```python
from build123d import *

# Parameters (mm, degrees)
SKETCH2_W             = 67.071067812
SKETCH2_H             = 337.071067812
SKETCH2_W_2           = 60
SKETCH2_H_2           = 330
BOSS_EXTRUDE1_DEPTH   = 12.5
SKETCH3_W             = 67.071067812
SKETCH3_H             = 337.071067812
BOSS_EXTRUDE2_DEPTH   = 5
BODY_MOVE_COPY2_ANGLE = 180
BOSS_EXTRUDE3_DEPTH   = 5


with BuildPart() as part:
    # Sketch2 → Boss-Extrude1 (new body)
    with BuildSketch(Plane(origin=(0, 0, 0), x_dir=(1, 0, 0), z_dir=(0, 1, 0))):
        with Locations((30, 165)):
            Rectangle(SKETCH2_W, SKETCH2_H)
        with Locations((30, 165)):
            Rectangle(SKETCH2_W_2, SKETCH2_H_2, mode=Mode.SUBTRACT)
    extrude(amount=BOSS_EXTRUDE1_DEPTH)

    # Sketch3 → Boss-Extrude2 (add)
    with BuildSketch(Plane.XZ):
        with Locations((30, -165)):
            Rectangle(SKETCH3_W, SKETCH3_H)
    extrude(amount=BOSS_EXTRUDE2_DEPTH)


with BuildPart() as body_2:
    # Split1: the piece on the far side of the plane
    add(part.part)
    split(bisect_by=Plane(origin=(0, 0, -165), x_dir=(-1, 0, 0), z_dir=(0, 0, -1)), keep=Keep.BOTTOM)


with BuildPart() as part_1:
    add(part.part)

    # Split1
    split(bisect_by=Plane(origin=(0, 0, -165), x_dir=(-1, 0, 0), z_dir=(0, 0, -1)), keep=Keep.TOP)

    # Sketch4 → Boss-Extrude3 (add)
    with BuildSketch(Plane.XY.offset(-165)):
        Polygon((60, 0), (0, 0), (0, 12.5), (-3.535533906, 12.5), (-3.535533906, -5), (63.535533906, -5), (63.535533906, 12.5), (60, 12.5), align=None)
    extrude(amount=BOSS_EXTRUDE3_DEPTH)


with BuildPart() as body_2_1:
    # Body-Move/Copy2: read off the stored shape, not the designer's step
    # Body-Move/Copy2: moved
    add(body_2.part.moved(Location((-127.0710678, -25, 0))).rotate(Axis((0, 0, 0), (0, 0, 1)), BODY_MOVE_COPY2_ANGLE))


solid = part_1.part
```
Check sheet for the modelled part. Datum: model origin and axes. Units: mm. A direction names the side the tool comes from. Give positions to 0.01 mm unless a question says otherwise; leave off trailing zeros. Write each loop counter-clockwise with the first axis right and the second up, starting at its lowest first coordinate (ties: lowest second). Pieces come first, ordered by that corner, then holes.
Item 1: Access from +Z, -Z, +X, -X, +Y, -Y to the whole of each face (thin tool, end or side, straight path). Record for faces 4 (the face through (0, 6, -246)), 5 (the face through (63.536, 4, -248)).
Item 2: Gauge pin test, flat ends, axial feed: pin 1 (5 mm diameter, centred on x = 16.5, y = 6.5, fed in from +Z); pin 2 (8 mm diameter, centred on x = 16.5, z = -186, fed in from +Y). Record the tip position at first contact, or that the pin passes through.
Item 3: Cross-section at B-B (z = -311). Enter the section's corners in (x, y).
Item 4: Cross-section at A-A (y = 8). Enter the section's corners in (x, z), and give its area (3 significant figures).
Item 5: Draft check along X on faces 1 (the face through (-3.536, 4, -248)), 2 (the face through (60, 6, -246)), 3 (the face through (22, -2, -160)). Enter one of: released by +X, released by -X, zero draft, split by the parting line, or undercut.
Item 6: Scan lines: L1, parallel to X at y = 4, z = -319; L2, parallel to Y at x = 59.5, z = -177; L3, parallel to Z at x = 19, y = 6.5. Record each from-to range of solid material in increasing order.
Item 7: Cross-section at C-C (x = 43.5). Enter the section's corners in (y, z).
Report:
1. face 4: +Z, +Y
1. face 5: +Z, -Z, +X, +Y, -Y
2. pin 1: stops at z = -330
2. pin 2: stops at y = 0
3. outline: (-3.54, -5) - (63.54, -5) - (63.54, 12.5) - (60, 12.5) - (60, 0) - (0, 0) - (0, 12.5) - (-3.54, 12.5) - close
4. outline: (-3.54, -333.54) - (63.54, -333.54) - (63.54, -160) - (60, -160) - (60, -330) - (0, -330) - (0, -160) - (-3.54, -160) - close
4. area: 1,440 mm2
5. face 1: released by -X
5. face 2: undercut
5. face 3: zero draft
6. L1: x = -3.54 to 0, 60 to 63.54
6. L2: y = -5 to 0
6. L3: z = -333.54 to -330
7. outline: (-5, -333.54) - (12.5, -333.54) - (12.5, -330) - (0, -330) - (0, -160) - (-5, -160) - close
